Geometry: final body of the model. Coordinates: model frame, mm. A direction names the side the tool comes from. Round coordinates to 2 decimals unless told otherwise and drop trailing zeros. Loops run counter-clockwise (first coordinate to the right, second up) from the corner with the lowest first, then second, coordinate; pieces in that order, holes last. Notation, with made-up numbers: M 33.25,-3.5 L 60.25,-3.5 A13 ccw 60.25,20.5 Z; hole C -18,-21.75 d9. An arc over 180 degrees is marked long. Return JSON: item names as keys, results as strings.
from build123d import *

# Parameters (mm, degrees)
F0_W     = 209.296
F0_H     = 133.096
F1_DEPTH = 2.9972
F2_W     = 25.273
F2_H     = 25.4
F3_DEPTH = 0.254


with BuildPart() as f1:
    # F0 (on Top) → F1 (new body)
    with BuildSketch(Plane.XY):
        Rectangle(F0_W, F0_H)
    extrude(amount=F1_DEPTH)

    # F2 (on face) → F3 (join)
    with BuildSketch(Plane.XY.offset(2.9972)):
        Polygon((-47.498, 66.548), (-50.673, 66.548), (-50.673, 12.7), (-104.648, 12.7), (-104.648, 9.525), (-22.225, 9.525), (-22.225, -66.548), (-19.05, -66.548), (-19.05, 66.548), (-22.225, 66.548), (-22.225, 41.275), (-47.498, 41.275), align=None)
        with Locations((-34.8615, 25.4)):
            Rectangle(F2_W, F2_H, mode=Mode.SUBTRACT)
    extrude(amount=F3_DEPTH)


solid = f1.part
Q1. Reachability of faces 1 (the flat face through (-35, 54, 2.997)), 2 (the flat face through (-64, -28, 2.997)), 3 (the flat face through (42, 1, 2.997)), 4 (the flat face through (-1, 1, 0)), 5 (the flat face through (-78, 40, 2.997)) from +Z, -Z, +X, -X, +Y, -Y: full face, straight path, thin tool, end or side. Return the list, or none.
Determined:
{"face 1": "+Z, +Y", "face 2": "+Z, -X, -Y", "face 3": "+Z, +X, +Y, -Y", "face 4": "-Z, +X, -X, +Y, -Y", "face 5": "+Z, -X, +Y"}
Q2. Material intervals for L1, parallel to Z at x = 36.5, y = 57, sorted ascending.
Determined:
{"L1": "z = 0 to 3"}
Q3. Pin query (flat end, axial travel): pin 1 (2 mm diameter, centred on x = -8.5, y = -27, fed in from +Z). Return the tip coordinate at first contact, or that it passes through.
Determined:
{"pin 1": "stops at z = 3"}
Q4. Section query B-B (y = 46.5). Output: boundary loops of the cut face in (x, z) (3 decimals), plus the area to 3 significant figures.
Determined:
{"outline": "M -104.648,0 L 104.648,0 L 104.648,2.997 L -19.05,2.997 L -19.05,3.251 L -22.225,3.251 L -22.225,2.997 L -47.498,2.997 L -47.498,3.251 L -50.673,3.251 L -50.673,2.997 L -104.648,2.997 Z", "area": "629 mm^2"}
Q5. Section query D-D (x = 89.5). Output: boundary loops of the cut face in (y, z).
Determined:
{"outline": "M -66.55,0 L 66.55,0 L 66.55,3 L -66.55,3 Z"}
Q6. Pull-direction query (Y, two-part tool) for faces 6 (the flat face through (-43, 10, 3.251)), 7 (the flat face through (-35, 26, 2.997)); classes: pulls with the +Y half, pulls with the -Y half, needs draft (parallel to the pull), parting line crosses it, or undercut.
Determined:
{"face 6": "needs draft", "face 7": "undercut"}
Q7. Section query C-C (y = -54.5). Output: boundary loops of the cut face in (x, z) (3 decimals).
Determined:
{"outline": "M -104.648,0 L 104.648,0 L 104.648,2.997 L -19.05,2.997 L -19.05,3.251 L -22.225,3.251 L -22.225,2.997 L -104.648,2.997 Z"}
Q8. Section query A-A (x = -75.5). Output: boundary loops of the cut face in (y, z) (3 decimals), plus the area to 3 significant figures.
Determined:
{"outline": "M -66.548,0 L 66.548,0 L 66.548,2.997 L 12.7,2.997 L 12.7,3.251 L 9.525,3.251 L 9.525,2.997 L -66.548,2.997 Z", "area": "400 mm^2"}
